from build123d import *

# Parameters (mm, degrees)
POCKET_DEPTH    = 13
SKETCH002_R     = 1.7
POCKET001_DEPTH = 17
POCKET002_DEPTH = 1.5
SKETCH004_R     = 5
POCKET003_DEPTH = 18.001
SKETCH005_R     = 8.2
POCKET004_DEPTH = 9
SKETCH006_W     = 30.6
SKETCH006_H     = 7
POCKET005_DEPTH = 4
SKETCH007_R     = 1.7
POCKET006_DEPTH = 14.001
POCKET007_DEPTH = 11
POCKET008_DEPTH = 247.121056
SKETCH010_R     = 1.7
POCKET009_DEPTH = 18.001
SKETCH011_R     = 2.95
POCKET010_DEPTH = 3


with BuildPart() as part:
    # Sketch → Revolution (revolve)
    with BuildSketch(Plane.XZ):
        Polygon((0, 18), (37, 18), (37, 3), (40, 3), (40, 0), (0, 0), align=None)
    revolve(axis=Axis((0, 0, 0), (0, 0, 1)))

    # Sketch001 (on Face5 of Revolution) → Pocket (cut)
    with BuildSketch(Plane(origin=(0, 0, 0), x_dir=(1, 0, 0), z_dir=(0, 0, -1))):
        Polygon((-11.5, -19.5), (11.5, -19.5), (11.5, -23), (5, -29.5), (5, -54.5), (2.5, -54.5), (2.5, -29.5), (9, -23), (-9, -23), (-2.5, -29.5), (-2.5, -54.5), (-5, -54.5), (-5, -29.5), (-11.5, -23), align=None)
    extrude(amount=-POCKET_DEPTH, mode=Mode.SUBTRACT)

    # Sketch002 (on DatumPlane) → Pocket001 (cut)
    with BuildSketch(Plane.XZ.offset(-40)):
        with Locations((0, 6.5)):
            Circle(SKETCH002_R)
    extrude(amount=POCKET001_DEPTH, mode=Mode.SUBTRACT)

    # Sketch003 (on DatumPlane) → Pocket002 (cut, symmetric)
    with BuildSketch(Plane.XZ.offset(-25.85)):
        Polygon((0, 9.85), (-2.901185, 8.175), (-2.901185, -1.825), (2.901185, -1.825), (2.901185, 8.175), align=None)
    extrude(amount=POCKET002_DEPTH, both=True, mode=Mode.SUBTRACT)

    # Sketch004 (on Face1 of Pocket002) → Pocket003 (cut, through all)
    with BuildSketch(Plane(origin=(0, 0, 18), x_dir=(-1, 0, 0), z_dir=(0, 0, 1))):
        Circle(SKETCH004_R)
    extrude(amount=-POCKET003_DEPTH, mode=Mode.SUBTRACT)

    # Sketch005 (on Face12 of Pocket003) → Pocket004 (cut)
    with BuildSketch(Plane(origin=(0, 0, 0), x_dir=(1, 0, 0), z_dir=(0, 0, -1))):
        Circle(SKETCH005_R)
    extrude(amount=-POCKET004_DEPTH, mode=Mode.SUBTRACT)

    # Sketch006 (on Face14 of Pocket004) → Pocket005 (cut)
    with BuildSketch(Plane(origin=(0, 0, 0), x_dir=(1, 0, 0), z_dir=(0, 0, -1))):
        Rectangle(SKETCH006_W, SKETCH006_H)
    extrude(amount=-POCKET005_DEPTH, mode=Mode.SUBTRACT)

    # Sketch007 (on Face39 of Pocket005) → Pocket006 (cut, through all)
    with BuildSketch(Plane(origin=(0, 0, 4), x_dir=(1, 0, 0), z_dir=(0, 0, -1))):
        with Locations((-11, 0)):
            Circle(SKETCH007_R)
        with Locations((11, 0)):
            Circle(SKETCH007_R)
    extrude(amount=-POCKET006_DEPTH, mode=Mode.SUBTRACT)

    # Sketch008 (on Face1 of Pocket006) → Pocket007 (cut)
    with BuildSketch(Plane(origin=(0, 0, 18), x_dir=(-1, 0, 0), z_dir=(0, 0, 1))):
        Polygon((11, 3.35), (8.098815, 1.675), (8.098815, -1.675), (11, -3.35), (13.901185, -1.675), (13.901185, 1.675), align=None)
        Polygon((-11, 3.35), (-13.901185, 1.675), (-13.901185, -1.675), (-11, -3.35), (-8.098815, -1.675), (-8.098815, 1.675), align=None)
    extrude(amount=-POCKET007_DEPTH, mode=Mode.SUBTRACT)

    # Sketch009 (on Face29 of Pocket007) → Pocket008 (cut, through all)
    with BuildSketch(Plane(origin=(0, 0, 0), x_dir=(1, 0, 0), z_dir=(0, 0, -1))):
        with BuildLine():
            ThreePointArc((16.792662, -2.646981), (14.722432, 8.5), (6.103978, 15.866362))
            ThreePointArc((4.890242, 18.250631), (5.039745, 16.82567), (6.103978, 15.866362))
            Line((4.890242, 18.250631), (7.747298, 28.913308))
            ThreePointArc((10.324426, 30.288715), (8.737473, 30.160109), (7.747298, 28.913308))
            ThreePointArc((31.393009, -6.203142), (27.712813, 16), (10.324426, 30.288715))
            ThreePointArc((28.913308, -7.747298), (30.488157, -7.513181), (31.393009, -6.203142))
            Line((18.250631, -4.890242), (28.913308, -7.747298))
            ThreePointArc((16.792662, -2.646981), (17.091331, -4.048288), (18.250631, -4.890242))
        make_face()
    pocket008 = extrude(amount=-POCKET008_DEPTH, mode=Mode.SUBTRACT)

    # Mirrored: Pocket008 across Sketch009 V_Axis
    add(pocket008.mirror(Plane(origin=(0, 0, 0), x_dir=(0, 0, -1), z_dir=(1, 0, 0))), mode=Mode.SUBTRACT)

    # Sketch010 (on Face43 of Mirrored) → Pocket009 (cut, through all)
    with BuildSketch(Plane(origin=(0, 0, 0), x_dir=(1, 0, 0), z_dir=(0, 0, -1))):
        with Locations((0, 18)):
            Circle(SKETCH010_R)
        with Locations((-16, -13)):
            Circle(SKETCH010_R)
        with Locations((16, -13)):
            Circle(SKETCH010_R)
    extrude(amount=-POCKET009_DEPTH, mode=Mode.SUBTRACT)

    # Sketch011 (on Face43 of Pocket009) → Pocket010 (cut)
    with BuildSketch(Plane(origin=(0, 0, 0), x_dir=(1, 0, 0), z_dir=(0, 0, -1))):
        with Locations((0, 18)):
            Circle(SKETCH011_R)
        with Locations((16, -13)):
            Circle(SKETCH011_R)
        with Locations((-16, -13)):
            Circle(SKETCH011_R)
    extrude(amount=-POCKET010_DEPTH, mode=Mode.SUBTRACT)


solid = part.part
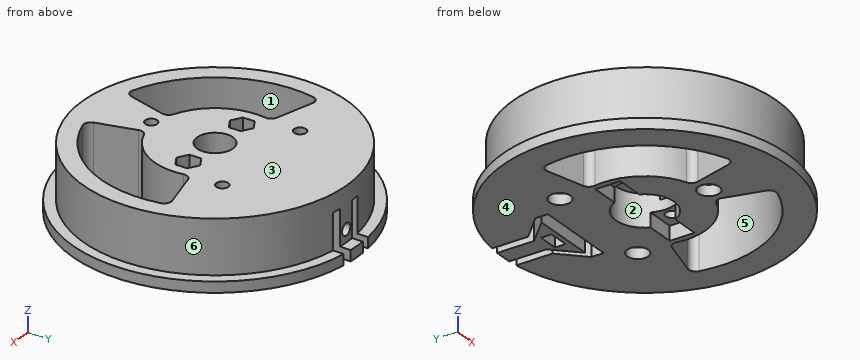
Source: CAD feature listing. Evaluate the final solid. Frame: model axes, mm. Face numbers are marked on the shaded views. A direction names the side the tool comes from. Coordinates: 2 decimals unless noted, no trailing zeros. Loops run counter-clockwise (first coordinate to the right, second up) from the corner with the lowest first, then second, coordinate; pieces in that order, holes last. Notation, with made-up numbers: (-22, -33.75) -> (13, -33.75) arc R7 ccw to (13, -23.75) -> close; hole circle Ø1 at (26.25, -32.75). An arc over 180 degrees is marked (long way). Answer in a Markdown table with one row per item. Add a question column.
Q1. Section B-B on x = -20. Return the cut outline in (y, z).
Q2. Section D-D on y = -14. Return the cut outline in (x, z), and give its area (3 significant figures).
Q3. Ray query, line 1 along X through (y, z) = (0, 2); line 2 along Y through (x, z) = (0, 4); line 3 along X through (y, z) = (2.5, 1.75). Return the intervals inside material, ascending.
Q4. Section C-C on z = 14.25. Give the number of separate pieces and of enclosed holes in the cut face, and give its area (3 significant figures).
Q5. Contact query for flat-ended pins moving along their axis: pin 1 Ø1.2 at (x, z) = (10, 2.5) entering from +Y; pin 2 Ø5.5 at (x, y) = (11, 0) entering from +Z; pin 3 Ø4.5 at (x, y) = (-11, 0) entering from -Z. Output: stop coordinate, or through.
Q6. Pull-direction query (X, two-part tool) for the marked faces 4, 5 and 6; classes: pulls with the +X half, pulls with the -X half, needs draft (parallel to the pull), parting line crosses it, or undercut.
Q7. Section A-A on y = 13. Return the cut outline in (x, z), and give its area (3 significant figures).
Q8. Reachability of the marked faces 1, 2 and 3 from +Z, -Z, +X, -X, +Y, -Y: full face, straight path, thin tool, end or side. Return the list, or none.
Computed values:
| question | item | result |
|---|---|---|
| 1 | outline | (-34.64, 0) -> (-24.98, 0) -> (-24.98, 18) -> (-31.13, 18) -> (-31.13, 3) -> (-34.64, 3) -> close; (5.36, 0) -> (34.64, 0) -> (34.64, 3) -> (31.13, 3) -> (31.13, 18) -> (5.36, 18) -> close |
| 2 | outline | (-37.47, 0) -> (-28.77, 0) -> (-28.77, 18) -> (-34.25, 18) -> (-34.25, 3) -> (-37.47, 3) -> close; (-9.64, 0) -> (9.64, 0) -> (9.64, 18) -> (-9.64, 18) -> close; (28.77, 0) -> (37.47, 0) -> (37.47, 3) -> (34.25, 3) -> (34.25, 18) -> (28.77, 18) -> close |
| 2 | area | 564 mm^2 |
| 3 | line 1 | x = -40 to -32, -17 to -15.3, 15.3 to 17, 32 to 40 |
| 3 | line 2 | y = -37 to -19.7, -16.3 to -8.2, 8.2 to 19.5, 23 to 24.35, 27.35 to 37 |
| 3 | line 3 | x = -39.92 to -31.9, -16.82 to -15.3, 15.3 to 16.82, 31.9 to 39.92 |
| 4 | separate pieces | 1 |
| 4 | enclosed holes | 8 |
| 4 | area | 2,990 mm^2 |
| 5 | pin 1 | stops at y = 38.88 |
| 5 | pin 2 | stops at z = 7 |
| 5 | pin 3 | stops at z = 4 |
| 6 | face 4 | needs draft |
| 6 | face 5 | undercut |
| 6 | face 6 | parting line crosses it |
| 7 | outline | (-37.83, 0) -> (-18.95, 0) -> (-18.95, 3) -> (-17.7, 3) -> (-17.7, 18) -> (-34.64, 18) -> (-34.64, 3) -> (-37.83, 3) -> close; (-14.3, 3) -> (-13.05, 3) -> (-13.05, 0) -> (13.05, 0) -> (13.05, 3) -> (14.3, 3) -> (14.3, 18) -> (-14.3, 18) -> close; (17.7, 3) -> (18.95, 3) -> (18.95, 0) -> (37.83, 0) -> (37.83, 3) -> (34.64, 3) -> (34.64, 18) -> (17.7, 18) -> close |
| 7 | area | 1,130 mm^2 |
| 8 | face 1 | +Z, -Z |
| 8 | face 2 | -Z |
| 8 | face 3 | +Z, +X, -X, +Y, -Y |
